from build123d import *

# Parameters (mm, degrees)
BOSS_EXTRUDE1_DEPTH = 130
SKETCH2_R           = 1.9
CUT_EXTRUDE1_DEPTH  = 261.334886359


with BuildPart() as part:
    # Sketch1 → Boss-Extrude1 (new, symmetric)
    with BuildSketch(Plane.XY):
        Polygon((0, 0), (0, -1.382978723), (10, -1.382978723), (10, 8.617021277), (3.448211747, 8.617021277), (3, 8.117021277), (3, 6.617021277), (7.587018089, 6.617021277), (7.587018089, 5.117021277), (3, 0), align=None)
    boss_extrude1 = extrude(amount=BOSS_EXTRUDE1_DEPTH, both=True)

    # Mirror1: Boss-Extrude1 across plane
    add(boss_extrude1.mirror(Plane(origin=(0, 0, 0), x_dir=(0, 0, 1), z_dir=(1, 0, 0))))

    # Sketch2 → Cut-Extrude1 (cut, through all)
    with BuildSketch(Plane.XY.offset(130)):
        with Locations((7.646716257, 0.97030502)):
            Circle(SKETCH2_R)
    cut_extrude1 = extrude(amount=-CUT_EXTRUDE1_DEPTH, mode=Mode.SUBTRACT)

    # Mirror2: Cut-Extrude1 across plane
    add(cut_extrude1.mirror(Plane(origin=(0, 0, 0), x_dir=(0, 0, 1), z_dir=(1, 0, 0))), mode=Mode.SUBTRACT)


solid = part.part
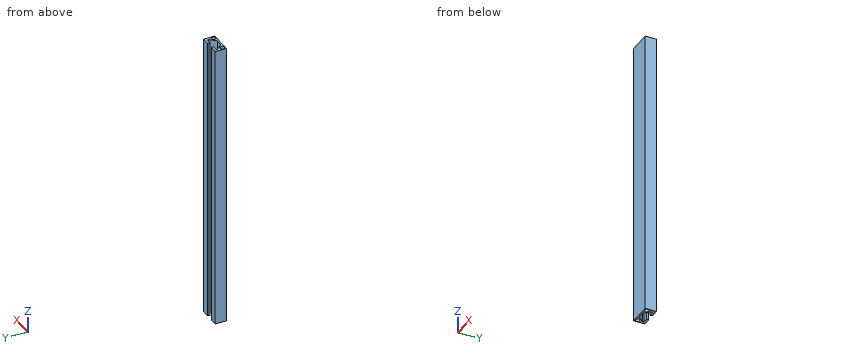
Geometry check sheet. Reference: the model listing, model coordinates, mm. Coordinates: 2 decimals unless noted, no trailing zeros. Order: outer loops, then holes, each group sorted by start corner. A loop starts at its lowest first (then second) coordinate and runs counter-clockwise, first axis right, second up. Notation, with made-up numbers: (-19.5, 79.25) - (-8.5, 79.25) arc R12 cw to (-8.5, 89.25) - close; hole circle Ø7 at (73, 70.5). An arc over 180 degrees is marked (long way). Answer in a Markdown table with one row per item. Add a question column.
1) Cross-section at A-A, the plane z = 7. Record the cut outline in (x, y).
2) Cross-section at B-B, the plane x = 0.25. Record the cut outline in (y, z), then the cut area to 3 significant figures.
3) Gauge pin test, flat ends, axial feed: P1, Ø4, axis at x = -1, y = 5, coming from the -Z side; P2, Ø6.5, axis at x = -0.5, z = 2, coming from the +Y side. Record the tip position at first contact, or that the pin passes through.
4) Material ranges on line 1 along X through (y, z) = (-0.5, 64.5); line 2 along X through (y, z) = (2.25, 12); line 3 along Y through (x, z) = (-6.75, 67), recorded low to high. Write a range as [from, to].
Check result:
| question | item | result |
|---|---|---|
| 1 | outline | (-10, -1.38) - (10, -1.38) - (10, 8.62) - (3.45, 8.62) - (3, 8.12) - (3, 6.62) - (7.59, 6.62) - (7.59, 5.12) - (3, 0) - (-3, 0) - (-7.59, 5.12) - (-7.59, 6.62) - (-3, 6.62) - (-3, 8.12) - (-3.45, 8.62) - (-10, 8.62) - close; hole circle Ø3.8 at (-7.65, 0.97); hole circle Ø3.8 at (7.65, 0.97) |
| 2 | outline | (-1.38, -130) - (0, -130) - (0, 130) - (-1.38, 130) - close |
| 2 | area | 360 mm² |
| 3 | P1 | passes through |
| 3 | P2 | stops at y = 8.62 |
| 4 | line 1 | x = [-10, -8.85], [-6.44, 6.44], [8.85, 10] |
| 4 | line 2 | x = [-10, -9.05], [-6.24, -5.02], [5.02, 6.24], [9.05, 10] |
| 4 | line 3 | y = [-1.38, -0.7], [2.65, 4.18], [6.62, 8.62] |
